The listing builds one solid part. Answer for the finished solid, in the listing's coordinates (mm). A direction names the side the tool comes from. Round coordinates to 2 decimals unless told otherwise and drop trailing zeros. Order: outer loops, then holes, each group sorted by start corner. A loop starts at its lowest first (then second) coordinate and runs counter-clockwise, first axis right, second up. Notation, with made-up numbers: (42, 7.25) - (60, 7.25) arc R35 cw to (60, 42.25) - close; hole circle Ø9 at (-16.5, -14.75). An arc over 180 degrees is marked (long way). One line per item, written item: value. Start each with the question number.
1. Section C-C, the plane y = -29.5 is taken. Give the vertices of the cut face in (x, z), then the cut area to 3 significant figures.
2. Flat-ended cylindrical pins translate along their axes: P1, Ø12, axis at x = 118.5, z = 61, coming from the +Y side; P2, Ø12, axis at y = -93.5, z = 41, coming from the +X side; P3, Ø1.8, axis at y = 2, z = 53, coming from the +X side. Find the tip coordinate at first contact, or state that the pin passes through.
3. A tool of negligible diameter and unlimited length cuts with its end or side. For faces 4 (the flat face through (97, 3, 39)), 5 (the flat face through (0, -124, 39)), 6 (the flat face through (-2, -155, 80)), from which of +Z, -Z, +X, -X, +Y, -Y can it reach the whole face along a straight path? Write none if from no direction.
4. Section D-D, the plane z = 13 is taken. Give the vertices of the cut face in (x, y).
5. Section B-B, the plane x = 85 is taken. Give the vertices of the cut face in (y, z).
6. For a pull along Y with two mould halves and no side action, classify faces 1 (the flat face through (197, -255, 39)), 2 (the flat face through (103, -258, 39)), 3 (the cylindrical face through (-3.042, -239.983, 55.769)) as released by +Y, released by -Y, zero draft, split by the parting line, or undercut.
7. Straight lines are drawn through the part: line 1 (Y direction, x = 26.5, z = 53.5); line 2 (Z direction, x = -1.55, y = -29.5); line 3 (Y direction, x = -3.8, z = 55). For each, find the intervals that lie inside material, in ascending order.
8. Section A-A, the plane z = 55 is taken. Give the vertices of the cut face in (x, y), then the cut area to 3 significant figures.
from build123d import *

# Parameters (mm, degrees)
SM_BASE_FLANGE_1_DEPTH = 80
SKETCH_6_R             = 17.5
CUT_EXTRUDE_1_DEPTH    = 10


# Sheet-metal steps are written as plain solids
with BuildPart() as part:
    # Sketch 1 → 基体-法兰1 (new body)
    with BuildSketch(Plane.XY):
        with BuildLine():
            Line((97, 0), (6, 0))
            ThreePointArc((6, 0), (1.757359313, -1.757359313), (0, -6))
            Line((0, -6), (0, -246))
            ThreePointArc((0, -246), (1.757359313, -250.242640687), (6, -252))
            Line((6, -252), (197, -252))
            Line((197, -252), (197, -258))
            Line((197, -258), (6, -258))
            ThreePointArc((6, -258), (-2.485281374, -254.485281374), (-6, -246))
            Line((-6, -246), (-6, -6))
            ThreePointArc((-6, -6), (-2.485281374, 2.485281374), (6, 6))
            Line((6, 6), (97, 6))
            Line((97, 6), (97, 0))
        make_face()
    extrude(amount=SM_BASE_FLANGE_1_DEPTH)

    # 草图6 → 切除-拉伸1 (cut)
    with BuildSketch(Plane(origin=(-6, 0, 0), x_dir=(0, 0, -1), z_dir=(1, 0, 0))):
        with Locations(Location((-55, -29.5, 0), (0, 0, 90))):
            Circle(SKETCH_6_R)
        with Locations(Location((-55, -222.5, 0), (0, 0, 90))):
            Circle(SKETCH_6_R)
    extrude(amount=CUT_EXTRUDE_1_DEPTH, mode=Mode.SUBTRACT)


solid = part.part
Answer list:
1. outline: (-6, 0) - (0, 0) - (0, 37.5) - (-6, 37.5) - close; (-6, 72.5) - (0, 72.5) - (0, 80) - (-6, 80) - close
1. area: 270 mm²
2. P1: stops at y = -252
2. P2: stops at x = 0
2. P3: stops at x = 97
3. face 4: +Z, -Z, +X, +Y
3. face 5: +Z, -Z, +X
3. face 6: +Z, +X, -X, +Y, -Y
4. outline: (-6, -246) arc R12 ccw to (6, -258) - (197, -258) - (197, -252) - (6, -252) arc R6 cw to (0, -246) - (0, -6) arc R6 cw to (6, 0) - (97, 0) - (97, 6) - (6, 6) arc R12 ccw to (-6, -6) - close
5. outline: (-258, 0) - (-252, 0) - (-252, 80) - (-258, 80) - close; (0, 0) - (6, 0) - (6, 80) - (0, 80) - close
6. face 1: zero draft
6. face 2: released by -Y
6. face 3: undercut
7. line 1: y = -258 to -252, 0 to 6
7. line 2: z = 0 to 37.5, 72.5 to 80
7. line 3: y = -252.93 to -240, -205 to -47, -12 to 0.93
8. outline: (-6, -246) arc R12 ccw to (6, -258) - (197, -258) - (197, -252) - (6, -252) arc R6 cw to (0, -246) - (0, -240) - (-6, -240) - close; (-6, -205) - (0, -205) - (0, -47) - (-6, -47) - close; (-6, -12) - (0, -12) - (0, -6) arc R6 cw to (6, 0) - (97, 0) - (97, 6) - (6, 6) arc R12 ccw to (-6, -6) - close
8. area: 2,880 mm²
